Check sheet for the modelled part. Datum: model origin and axes. Units: mm. A direction names the side the tool comes from. Give positions to 0.01 mm unless a question says otherwise; leave off trailing zeros. Write each loop counter-clockwise with the first axis right and the second up, starting at its lowest first coordinate (ties: lowest second). Pieces come first, ordered by that corner, then holes. Notation, with made-up numbers: (21, 56.25) -> (66, 56.25) arc R22 ccw to (66, 77.25) -> close; hole circle Ø2 at (-19.5, 9). An arc over 180 degrees is marked (long way). Return JSON: item names as keys, results as strings.
from build123d import *

# Parameters (mm, degrees)
SKETCH1_W           = 10
SKETCH1_H           = 10
BOSS_EXTRUDE1_DEPTH = 11.5
CUT_EXTRUDE1_REACH  = 37.548
SKETCH2_R           = 3.25
SKETCH3_W           = 8.3
SKETCH3_H           = 1.55
BOSS_EXTRUDE2_DEPTH = 2.5
CUT_EXTRUDE2_REACH  = 55.761
SKETCH4_R           = 1


with BuildPart() as part:
    # Sketch1 → Boss-Extrude1 (new body)
    # profile 1 of 4: a face of its own
    with BuildSketch(Plane(origin=(0, 0, 0), x_dir=(1, 0, 0), z_dir=(0, 1, 0))):
        with BuildLine():
            Line((-27.472148501, 6.754381863), (-28.370678518, -4.662524505))
            Line((-28.370678518, -4.662524505), (-24.01063487, -4.662524505))
            Line((-24.01063487, -4.662524505), (-24.01063487, 5.337475495))
            Line((-24.01063487, 5.337475495), (-14.01063487, 5.337475495))
            Line((-14.01063487, 5.337475495), (-9.65, 6.907286969))
            Line((-9.65, 6.907286969), (-9.65, 9.407286969))
            Line((-9.65, 9.407286969), (-1.35, 9.407286969))
            Line((-1.35, 9.407286969), (-1.35, 6.907286969))
            Line((-1.35, 6.907286969), (9.65, 6.907286969))
            Line((9.65, 6.907286969), (14.01063487, 5.337475495))
            Line((14.01063487, 5.337475495), (24.01063487, 5.337475495))
            Line((24.01063487, 5.337475495), (24.01063487, -4.662524505))
            Line((24.01063487, -4.662524505), (28.370678518, -4.662524505))
            Line((28.370678518, -4.662524505), (27.472148501, 6.754381863))
            ThreePointArc((27.472148501, 6.754381863), (26.86214664, 8.165702195), (25.515789835, 8.908164787))
            Line((25.515789835, 8.908164787), (0, 13.407286969))
            Line((0, 13.407286969), (-11, 11.467690181))
            Line((-11, 11.467690181), (-25.515789835, 8.908164787))
            ThreePointArc((-25.515789835, 8.908164787), (-26.86214664, 8.165702195), (-27.472148501, 6.754381863))
        make_face()
    # profile 2 of 4: a face of its own
    with BuildSketch(Plane(origin=(0, 0, 0), x_dir=(1, 0, 0), z_dir=(0, 1, 0))):
        with Locations((-19.01063487, 0.337475495)):
            Rectangle(SKETCH1_W, SKETCH1_H)
        Polygon((-17.567259197, 2.837475495), (-16.123883525, 0.337475495), (-17.567259197, -2.162524505), (-20.454010543, -2.162524505), (-21.897386216, 0.337475495), (-20.454010543, 2.837475495), align=None, mode=Mode.SUBTRACT)
    # profile 3 of 4: a face of its own
    with BuildSketch(Plane(origin=(0, 0, 0), x_dir=(1, 0, 0), z_dir=(0, 1, 0))):
        Polygon((-11, 13.407286969), (-11, 11.467690181), (0, 13.407286969), align=None)
    # profile 4 of 4: a face of its own
    with BuildSketch(Plane(origin=(0, 0, 0), x_dir=(1, 0, 0), z_dir=(0, 1, 0))):
        with Locations((19.01063487, 0.337475495)):
            Rectangle(SKETCH1_W, SKETCH1_H)
        Polygon((20.454010543, 2.837475495), (21.897386216, 0.337475495), (20.454010543, -2.162524505), (17.567259197, -2.162524505), (16.123883525, 0.337475495), (17.567259197, 2.837475495), align=None, mode=Mode.SUBTRACT)
    extrude(amount=BOSS_EXTRUDE1_DEPTH)

    # Sketch2 → Cut-Extrude1 (cut, up to next)
    with BuildSketch(Plane(origin=(0, 0, -13.407286969), x_dir=(-1, 0, 0), z_dir=(0, 0, -1)), mode=Mode.PRIVATE) as cut_extrude1_sk1:
        with Locations((5.5, 5.75)):
            Circle(SKETCH2_R)
    cut_extrude1_tool1 = extrude(cut_extrude1_sk1.sketch, amount=-CUT_EXTRUDE1_REACH, mode=Mode.PRIVATE) & part.part
    add(cut_extrude1_tool1.solids().sort_by_distance((-5.5, 5.75, -13.407287))[0], mode=Mode.SUBTRACT)

    # Sketch3 → Boss-Extrude2 (add)
    with BuildSketch(Plane.XY.offset(-9.407286969)):
        with Locations((-5.5, 10.725)):
            Rectangle(SKETCH3_W, SKETCH3_H)
        with Locations((-5.5, 0.775)):
            Rectangle(SKETCH3_W, SKETCH3_H)
    extrude(amount=BOSS_EXTRUDE2_DEPTH)

    # Cut-Extrude2: up to this plane
    cut_extrude2_end = Plane(origin=(0, 11.5, 4.662524505), z_dir=(0, 0, -1))
    # Sketch4 → Cut-Extrude2 (cut, up to the surface)
    with BuildSketch(Plane(origin=(19.248080096, 0, -17.483724977), x_dir=(-0.6723668074346677, 0, -0.7402181274868325), z_dir=(0.7402181274868325, 0, -0.6723668074346677)), mode=Mode.PRIVATE) as cut_extrude2_sk1:
        with Locations((-16.853337608, 2)):
            Circle(SKETCH4_R)
    cut_extrude2_tool1 = split(extrude(cut_extrude2_sk1.sketch, amount=-CUT_EXTRUDE2_REACH, mode=Mode.PRIVATE), bisect_by=cut_extrude2_end, keep=Keep.BOTH, mode=Mode.PRIVATE)
    cut_extrude2 = cut_extrude2_tool1.solids().sort_by_distance((30.579705, 2, -5.008579))[0]
    add(cut_extrude2, mode=Mode.SUBTRACT)

    # Mirror1: Cut-Extrude2 across plane
    add(cut_extrude2.mirror(Plane(origin=(0, 0, 0), x_dir=(0, 0, 1), z_dir=(1, 0, 0))), mode=Mode.SUBTRACT)


solid = part.part
(1) Cross-section at B-B on x = -5.5. Enter the section's corners in (y, z).
Reply:
{"outline": "(0, -13.41) -> (2.5, -13.41) -> (2.5, -9.41) -> (1.55, -9.41) -> (1.55, -6.91) -> (0, -6.91) -> close; (9, -13.41) -> (11.5, -13.41) -> (11.5, -6.91) -> (9.95, -6.91) -> (9.95, -9.41) -> (9, -9.41) -> close"}
(2) Set-up check for faces 1 (the flat face through (16.835, 5.67, -1.57)), 2 (the flat face through (0, 11.5, -9)), 3 (the cylindrical face through (27, 6, -8)), 4 (the flat face through (14.011, 6, 0)), 5 (the flat face through (-1.35, 6, -8)): record each of +Z, -Z, +X, -X, +Y, -Y from which the full face is reachable in a straight line by a thin tool's end or side.
Reply:
{"face 1": "+Y, -Y", "face 2": "+Z, -Z, +X, -X, +Y", "face 3": "-Z, +X, +Y, -Y", "face 4": "+Z, +Y, -Y", "face 5": "+Z"}
(3) Depth check by flat-ended pin: pin 1 Ø3 at (x, y) = (-17.5, 9) entering from -Z; pin 2 Ø3 at (x, y) = (-19.5, 8) entering from -Z; pin 3 Ø0.8 at (y, z) = (7.5, -8) entering from +X; pin 4 Ø6 at (x, z) = (-10, 1.5) entering from -Y. Enter the tip coordinate at first touch or a pass-through.
Reply:
{"pin 1": "z = -10.59", "pin 2": "z = -10.23", "pin 3": "x = 27.24", "pin 4": "through"}
(4) Cross-section at C-C on z = -7.5. Enter the section's corners in (x, y).
Reply:
{"outline": "(-27.29, 0) -> (27.29, 0) -> (27.29, 11.5) -> (-27.29, 11.5) -> close; hole (-9.65, 1.55) -> (-1.35, 1.55) -> (-1.35, 9.95) -> (-9.65, 9.95) -> close"}
(5) Thickness scan on L1, parallel to Y at x = -5.5, z = -11.15; L2, parallel to X at y = 9.75, z = 3.75; L3, parallel to X at y = 7.75, z = -3. Record the ranges inside material, lowest first.
Reply:
{"L1": "0 to 2.5, 9 to 11.5", "L2": "-28.3 to -14.01, 14.01 to 28.3", "L3": "-27.77 to -14.01, 14.01 to 27.77"}
(6) Cross-section at A-A on y = 5.75. State how many separate pieces and enclosed holes the cut face has, then the cut area to 3 significant figures.
Reply:
{"separate pieces": "2", "enclosed holes": "2", "area": "472 mm^2"}
(7) Release check for a two-part mould opening along X. For faces 6 (the flat face through (19, 6, 2.163)), 7 (the cylindrical face through (-23.173, 2.3, 0.431)), 8 (the flat face through (12.937, 5.67, -11.126)), 9 (the flat face through (-21, 6, 4.663)) record: pulls with the +X half, pulls with the -X half, needs draft (parallel to the pull), parting line crosses it, or undercut.
Reply:
{"face 6": "undercut", "face 7": "undercut", "face 8": "pulls with the +X half", "face 9": "needs draft"}
